```python
from build123d import *

# Parameters (mm, degrees)
F0_R     = 42.7482
F1_DEPTH = 2.54
F2_R     = 39.5732
F3_DEPTH = 2.286
F4_R     = 13.208
F5_DEPTH = 4.827
F6_R     = 2.54


with BuildPart() as f1:
    # F0 (on Top) → F1 (new body)
    with BuildSketch(Plane.XY):
        Circle(F0_R)
    extrude(amount=F1_DEPTH)

    # F2 (on face) → F3 (join)
    with BuildSketch(Plane.XY.offset(2.54)):
        Circle(F2_R)
    extrude(amount=F3_DEPTH)

    # F4 (on face) → F5 (cut, through all)
    with BuildSketch(Plane.XY.offset(4.826)):
        Circle(F4_R)
    extrude(amount=-F5_DEPTH, mode=Mode.SUBTRACT)

    # F6
    f6_edges = [f1.edges().sort_by_distance(p)[0] for p in [
        (-13.208, 0, 0),
    ]]
    fillet(f6_edges, radius=F6_R)


solid = f1.part
```
The model under review builds one solid part; all positions refer to its coordinate system, in mm. A direction names the side the tool comes from. Round coordinates to 2 decimals unless told otherwise and drop trailing zeros. Order: outer loops, then holes, each group sorted by start corner. A loop starts at its lowest first (then second) coordinate and runs counter-clockwise, first axis right, second up. Notation, with made-up numbers: M -40,-38 L -29,-38 A17 ccw -29,-8 Z; hole C 15,-8 d11. An arc over 180 degrees is marked long. Use a Markdown table: item, result.
1) Consider section D-D (y = -26). Write out the cut boundary in (x, z).
Report:
| item | result |
|---|---|
| outline | M -33.93,0 L 33.93,0 L 33.93,2.54 L 29.83,2.54 L 29.83,4.83 L -29.83,4.83 L -29.83,2.54 L -33.93,2.54 Z |
2) Wall thickness on line 1 along Y through (x, z) = (0, 4); line 2 along Y through (x, z) = (11, 0.9); line 3 along X through (y, z) = (-3.5, 0.65): over which ranges is each line inside the solid? List them lowest first. Write a range as [from, to].
Report:
| item | result |
|---|---|
| line 1 | [-39.57, -13.21], [13.21, 39.57] |
| line 2 | [-41.31, -8.35], [8.35, 41.31] |
| line 3 | [-42.6, -13.61], [13.61, 42.6] |
3) Tool access review of faces 1 (the face through (17, 1, 4.826)), 2 (the face through (12, -38, 2.54)): name each direction out of +Z, -Z, +X, -X, +Y, -Y from which nothing blocks a thin tool from reaching the whole face with its end or side.
Report:
| item | result |
|---|---|
| face 1 | +Z, +X, -X, +Y, -Y |
| face 2 | +Z |
4) Consider section C-C (z = 1.6). Write out the cut boundary in (x, y), then the cut area to 3 significant figures.
Report:
| item | result |
|---|---|
| outline | C 0,0 d85.5; hole C 0,0 d26.78 |
| area | 5,180 mm^2 |
5) Insertion check: pin 1 (2 mm diameter, centred on x = -5, z = 2, fed in from +Y); pin 2 (1 mm diameter, centred on y = -28.5, z = 1, fed in from -X); pin 3 (2 mm diameter, centred on x = -9, z = 3, fed in from +Y). Each pin has a flat end and moves straight along its axis. Give the tip position at first contact, or say it passes through.
Report:
| item | result |
|---|---|
| pin 1 | y = 42.56 |
| pin 2 | x = -32.3 |
| pin 3 | y = 41.97 |
6) Draft analysis for pull direction X (two halves, no side actions). For faces 3 (the face through (18, 1, 0)), 4 (the face through (-8.58, -38.63, 3.67)), 5 (the face through (12.2, -5.06, 3.7)), state which applies: released by +X, released by -X, zero draft, split by the parting line, or undercut.
Report:
| item | result |
|---|---|
| face 3 | zero draft |
| face 4 | split by the parting line |
| face 5 | undercut |
7) Consider section A-A (y = 0). Write out the cut boundary in (x, z).
Report:
| item | result |
|---|---|
| outline | M -42.75,0 L -15.75,0 A2.54 ccw -13.21,2.54 L -13.21,4.83 L -39.57,4.83 L -39.57,2.54 L -42.75,2.54 Z; M 13.21,2.54 A2.54 ccw 15.75,0 L 42.75,0 L 42.75,2.54 L 39.57,2.54 L 39.57,4.83 L 13.21,4.83 Z |
